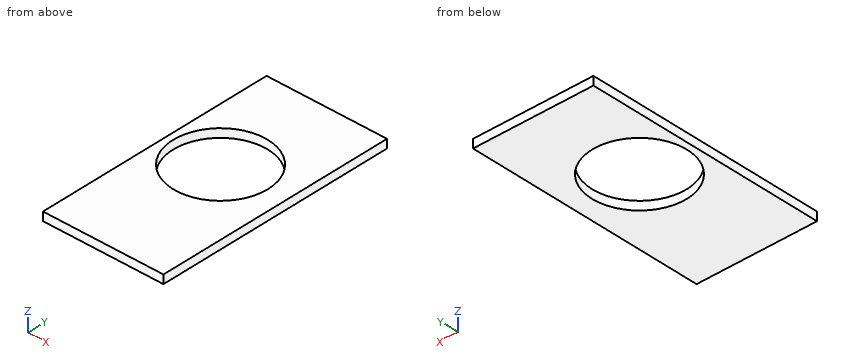
```python
from build123d import *

# Parameters (mm, degrees)
ESQUISSE1_W                  = 140
ESQUISSE1_H                  = 280
BOSS_EXTRU_1_DEPTH           = 10
ENL_V_MAT_EXTRU_1_DEPTH      = 314.209195267
ENL_V_MAT_EXTRU_1_DEPTH_BACK = 314.209195267
ESQUISSE2_R                  = 55


with BuildPart() as part:
    # Esquisse1 → Boss.-Extru.1 (new body)
    with BuildSketch(Plane.XY):
        with Locations((70, 140)):
            Rectangle(ESQUISSE1_W, ESQUISSE1_H)
    extrude(amount=BOSS_EXTRU_1_DEPTH)

    # Esquisse2 → Enlèv. mat.-Extru.1 (cut, two sides: drawn at the far end of the back side and taken through both)
    with BuildSketch(Plane.XY.offset(10).offset(-ENL_V_MAT_EXTRU_1_DEPTH_BACK)):
        with Locations((62.5, 155)):
            Circle(ESQUISSE2_R)
    extrude(amount=ENL_V_MAT_EXTRU_1_DEPTH + ENL_V_MAT_EXTRU_1_DEPTH_BACK, mode=Mode.SUBTRACT)


solid = part.part
```
Verification items for the finished model (mm, model axes). Round coordinates to 2 decimals unless told otherwise and drop trailing zeros. Order: outer loops, then holes, each group sorted by start corner. A loop starts at its lowest first (then second) coordinate and runs counter-clockwise, first axis right, second up. Notation, with made-up numbers: (81, 38.25) - (100, 38.25) arc R24 cw to (100, 58.25) - close; hole circle Ø6 at (78.5, 38). An arc over 180 degrees is marked (long way). Use CSV: the item, a comma, the result in double quotes. Start each with the question number.
1) Thickness scan on L1, parallel to X at y = 155, z = 2.25; L2, parallel to Y at x = 62.5, z = 4.5; L3, parallel to Y at x = 66, z = 9. Record the ranges inside material, lowest first.
2) Section check B-B, the plane y = 197. Record the cut outline in (x, z).
3) Section check A-A, the plane x = 62.5. Record the cut outline in (y, z), plus the area to 3 significant figures.
4) Go/stop test with a flat-tipped pin: P1, Ø2, axis at y = 161.5, z = 3, coming from the -X side. Record where the tip stops, or that it passes through.
Answers:
1,L1,"x = 0 to 7.5, 117.5 to 140"
1,L2,"y = 0 to 100, 210 to 280"
1,L3,"y = 0 to 100.11, 209.89 to 280"
2,outline,"(0, 0) - (26.99, 0) - (26.99, 10) - (0, 10) - close; (98.01, 0) - (140, 0) - (140, 10) - (98.01, 10) - close"
3,outline,"(0, 0) - (100, 0) - (100, 10) - (0, 10) - close; (210, 0) - (280, 0) - (280, 10) - (210, 10) - close"
3,area,"1,700 mm²"
4,P1,"stops at x = 0"
